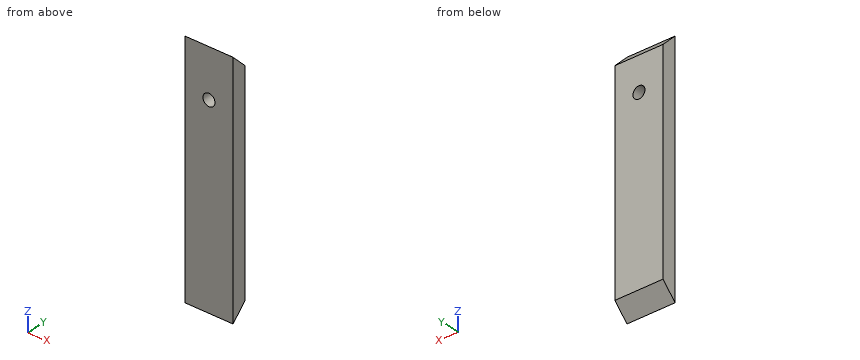
Autodesk Inventor part; units mm, degrees
ref_plane "YZ Plane" through (0, 0, 0) normal (1, 0, 0) x (0, 1, 0)
ref_plane "XZ Plane" through (0, 0, 0) normal (0, 1, 0) x (-1, 0, 0)
ref_plane "XY Plane" through (0, 0, 0) normal (0, 0, 1) x (1, 0, 0)
sketch "Skizze1" plane through (0, 0, 0) normal (0, 1, 0) x (-1, 0, 0)
  line L0 (35.9259, 133.0751) -> (-24.0741, 133.0751)
  line L1 (-24.0741, 133.0751) -> (-24.0741, -166.9249)
  line L2 (-24.0741, -166.9249) -> (35.9259, -166.9249)
  line L3 (35.9259, -166.9249) -> (35.9259, 133.0751)
  point P0 (0, 0)
  point P1 (5.9259, 83.0751)
  dimension "d0" = 60
  dimension "d1" = 300
  dimension "d24" = 30
  dimension "d25" = 50
extrude "Extrusion1" add sketch "Skizze1" along normal blind 18
chamfer "Fase1" distance 18 angle 45 1 edges at (-5.9259, 18, 133.0751)
chamfer "Fase2" distance 18 angle 45 1 edges at (-5.9259, 18, -166.9249)
sketch "Skizze4" plane through (0, 0, 0) normal (0, -1, 0) x (1, 0, 0)
  line L0 (-35.9259, -166.9249) -> (-35.9259, 133.0751)
  line L1 (-35.9259, 133.0751) -> (24.0741, 133.0751)
  point P0 (0, 0)
  point P1 (-5.9259, 73.0751)
  dimension "d33" = 30
  dimension "d34" = 60
hole "Bohrung5" at (-5.9259, 0, 73.0751) direction (0, 1, 0) diameter 15 end through all
sketch "Skizze2" plane through (0, 18, 0) normal (0, 1, 0) x (1, 0, 0)
  point P0 (38.0741, -40.5751)
sketch "Skizze3" plane through (0, 18, 0) normal (0, 1, 0) x (1, 0, 0)
  point P0 (38.0741, 74.4249)
properties part number "Front" material "Holz (Eiche)"
Source: CAD feature listing. Evaluate the final solid. Frame: model axes, mm. Coordinates: 2 decimals unless noted, no trailing zeros. Loops run counter-clockwise (first coordinate to the right, second up) from the corner with the lowest first, then second, coordinate; pieces in that order, holes last. Notation, with made-up numbers: M 31.5,26.25 L 49.5,26.25 A21 cw 49.5,52.25 Z; hole C 86.25,65.25 d7. An arc over 180 degrees is marked long. Answer in a Markdown table with one row per item.
Q1. First-contact query: pin 1 (12 mm diameter, centred on x = -24.5, z = 30.5, fed in from -Y); pin 2 (5 mm diameter, centred on x = -24.5, y = 15, fed in from +Z); pin 3 (3 mm diameter, centred on x = 17, y = 2.5, fed in from -Z). Flat tips, straight axial feed; report the tip coordinate or a pass-through.
Answers below:
| item | result |
|---|---|
| pin 1 | stops at y = 0 |
| pin 2 | stops at z = 120.58 |
| pin 3 | stops at z = -165.93 |
Q2. Section A-A on y = 5.75. Return the cut outline in (x, z).
Answers below:
| item | result |
|---|---|
| outline | M -35.93,-161.18 L 24.07,-161.18 L 24.07,127.33 L -35.93,127.33 Z; hole C -5.93,73.08 d15 |
Q3. Ray query, probe 1 along Z at (x, y) = (-3, 13.75); probe 2 along Z at (x, y) = (21.5, 6.25); probe 3 along Z at (x, y) = (0, 6). Return the intervals inside material, ascending. Write a range as from..to.
Answers below:
| item | result |
|---|---|
| probe 1 | z = -153.18..66.17, 79.98..119.33 |
| probe 2 | z = -160.68..126.83 |
| probe 3 | z = -160.93..68.48, 77.67..127.08 |
